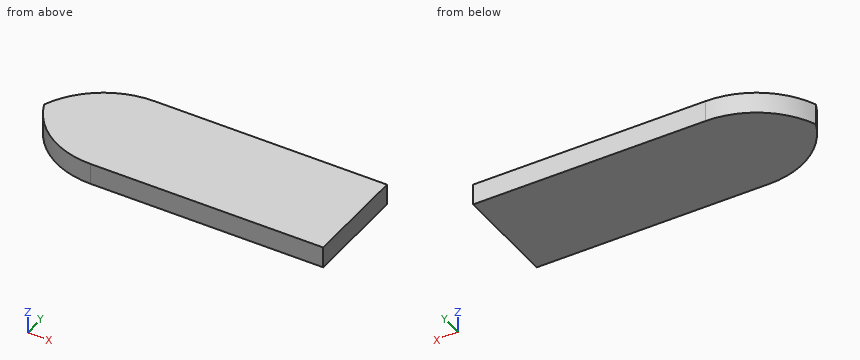
```python
from build123d import *

# Parameters (mm, degrees)
F0_W        = 75
F0_H        = 25
F1_DEPTH    = 5
F2_T1_DEPTH = 105


# Not quite as in the source:
# - a fillet or chamfer that OpenCascade refuses, or shapes differently, is made with other operations: its cross-section is extruded or revolved along the edge and cut away or added


with BuildPart() as f1:
    # F0 (on Top) → F1 (new body)
    with BuildSketch(Plane.XY):
        Rectangle(F0_W, F0_H)
    extrude(amount=F1_DEPTH)

    # F2: fillet of radius 20 on 2 edges, made by hand

    # F2_s2 → F2_t1 (cut)
    with BuildSketch(Plane.XY.offset(-50)):
        with BuildLine():
            ThreePointArc((-17.5, 12.5), (-31.6421356237, 6.6421356237), (-37.5, -7.5))
            Line((-37.5, -7.5), (-37.5, 12.5))
            Line((-37.5, 12.5), (-17.5, 12.5))
        make_face()
        with BuildLine():
            ThreePointArc((-37.5, 7.5), (-31.6421356237, -6.6421356237), (-17.5, -12.5))
            Line((-17.5, -12.5), (-37.5, -12.5))
            Line((-37.5, -12.5), (-37.5, 7.5))
        make_face()
    extrude(amount=F2_T1_DEPTH, mode=Mode.SUBTRACT)


solid = f1.part
```
Source: CAD feature listing. Evaluate the final solid. Frame: model axes, mm. Give positions to 0.01 mm unless a question says otherwise; leave off trailing zeros. Loops run counter-clockwise (first coordinate to the right, second up) from the corner with the lowest first, then second, coordinate; pieces in that order, holes last. Notation, with made-up numbers: (-33.5, 85.25) -> (18.5, 85.25) arc R30 cw to (18.5, 123.25) -> close; hole circle Ø3 at (18, 0.5). An arc over 180 degrees is marked (long way). Use a Markdown table: item, result. Add a question column.
(1) Ray query, line 1 (X direction, y = 6, z = 1.4); line 2 (X direction, y = 10.5, z = 3). Return the intervals inside material, ascending.
(2) First-contact query: pin 1 Ø1.5 at (y, z) = (-6.5, 4) entering from -X. Flat tip, straight axial feed; report the tip coordinate or a pass-through.
(3) Section query C-C (y = -4.5). Output: boundary loops of the cut face in (x, z), then the cut area to 3 significant figures.
(4) Section query A-A (x = -29.5). Output: boundary loops of the cut face in (y, z), then the cut area to 3 significant figures.
(5) Section query B-B (z = 4.3). Output: boundary loops of the cut face in (x, y), then the cut area to 3 significant figures.
Checked values:
| question | item | result |
|---|---|---|
| 1 | line 1 | -32.26 to 37.5 |
| 1 | line 2 | -26.22 to 37.5 |
| 2 | pin 1 | x = -32.48 |
| 3 | outline | (-33.5, 0) -> (37.5, 0) -> (37.5, 5) -> (-33.5, 5) -> close |
| 3 | area | 355 mm^2 |
| 4 | outline | (-8.5, 0) -> (8.5, 0) -> (8.5, 5) -> (-8.5, 5) -> close |
| 4 | area | 85.0 mm^2 |
| 5 | outline | (-36.04, 0) arc R20 ccw to (-17.5, -12.5) -> (37.5, -12.5) -> (37.5, 12.5) -> (-17.5, 12.5) arc R20 ccw to start |
| 5 | area | 1,710 mm^2 |
